Design review of the part built by this model. Coordinates are the model's own, in mm. A direction names the side the tool comes from. Coordinates: 2 decimals unless noted, no trailing zeros. Order: outer loops, then holes, each group sorted by start corner. A loop starts at its lowest first (then second) coordinate and runs counter-clockwise, first axis right, second up. Notation, with made-up numbers: M 48.25,20 L 57.25,20 A32 ccw 57.25,54 Z; hole C -36.5,-30.5 d9. An arc over 180 degrees is marked long. Answer in a Markdown table with one row per item.
from build123d import *

# Parameters (mm, degrees)
F_190_X_200_TRAY_FLOOR_SKETCH_W                       = 190
F_190_X_200_TRAY_FLOOR_SKETCH_H                       = 208
F_4_MM_TRAY_FLOOR_DEPTH                               = 4
ELECTRONICS_COMPARTMENT_WALL_SKETCH_W                 = 190
ELECTRONICS_COMPARTMENT_WALL_SKETCH_H                 = 175
ELECTRONICS_COMPARTMENT_WALL_SKETCH_W_2               = 176
ELECTRONICS_COMPARTMENT_WALL_SKETCH_H_2               = 161
F_22_MM_PERIMETER_WALLS_DEPTH                         = 22
F_3_2_START                                           = 17.2
EXTERNAL_WALL_CORD_GASKET_GROOVE_SKETCH_W             = 192
EXTERNAL_WALL_CORD_GASKET_GROOVE_SKETCH_H             = 177
EXTERNAL_WALL_CORD_GASKET_GROOVE_SKETCH_W_2           = 185.4
EXTERNAL_WALL_CORD_GASKET_GROOVE_SKETCH_H_2           = 170.4
F_3_2_HIGH_X_2_3_DEEP_EXTERNAL_PERIMETER_G_DEPTH      = 3.2
F_24_MM_GPS_ANTENNA_SHELF_SKETCH_W                    = 24
F_24_MM_GPS_ANTENNA_SHELF_SKETCH_H                    = 24
F_2_MM_GPS_ANTENNA_SHELF_DEPTH                        = 2
F_20_MM_GPS_ANTENNA_GUIDE_RING_SKETCH_W               = 24
F_20_MM_GPS_ANTENNA_GUIDE_RING_SKETCH_H               = 24
F_20_MM_GPS_ANTENNA_GUIDE_RING_SKETCH_W_2             = 20
F_20_MM_GPS_ANTENNA_GUIDE_RING_SKETCH_H_2             = 20
F_8_5_MM_GPS_ANTENNA_GUIDE_RING_DEPTH                 = 8.5
LEFT_GPS_ANTENNA_SNAP_LIP_SKETCH_W                    = 2.5
LEFT_GPS_ANTENNA_SNAP_LIP_SKETCH_H                    = 16
LEFT_GPS_ANTENNA_SNAP_LIP_DEPTH                       = 1.4
RIGHT_GPS_ANTENNA_SNAP_LIP_SKETCH_W                   = 2.5
RIGHT_GPS_ANTENNA_SNAP_LIP_SKETCH_H                   = 16
RIGHT_GPS_ANTENNA_SNAP_LIP_DEPTH                      = 1.4
F_190_MM_WIDE_ANGLED_DISPLAY_BULKHEAD_DEPTH           = 95
F_190_MM_WIDE_ANGLED_DISPLAY_BULKHEAD_DEPTH_BACK      = 95
F_92_X_58_MM_DISPLAY_OPENING_DEPTH                    = 46
F_92_X_58_MM_DISPLAY_OPENING_DEPTH_BACK               = 46
F_18_MM_FRONT_12_V_AND_SENSOR_HARNESS_PASS_DEPTH      = 40
F_18_MM_FRONT_12_V_AND_SENSOR_HARNESS_PASS_DEPTH_BACK = 40
F_18_MM_FRONT_HARNESS_GROMMET_SKETCH_R                = 9
LEFT_SCREEN_HOLDER_CORNER_CHAMFER_DEPTH               = 110
LEFT_SCREEN_HOLDER_CORNER_CHAMFER_DEPTH_BACK          = 110
RIGHT_SCREEN_HOLDER_CORNER_CHAMFER_DEPTH              = 110
RIGHT_SCREEN_HOLDER_CORNER_CHAMFER_DEPTH_BACK         = 110


with BuildPart() as part:
    # 190 x 200 Tray Floor Sketch → 4 mm Tray Floor (new body)
    with BuildSketch(Plane.XY):
        with Locations((0, 96)):
            Rectangle(F_190_X_200_TRAY_FLOOR_SKETCH_W, F_190_X_200_TRAY_FLOOR_SKETCH_H)
    extrude(amount=F_4_MM_TRAY_FLOOR_DEPTH)

    # Electronics Compartment Wall Sketch → 22 mm Perimeter Walls (add)
    with BuildSketch(Plane.XY):
        with Locations((0, 112.5)):
            Rectangle(ELECTRONICS_COMPARTMENT_WALL_SKETCH_W, ELECTRONICS_COMPARTMENT_WALL_SKETCH_H)
        with Locations((0, 112.5)):
            Rectangle(ELECTRONICS_COMPARTMENT_WALL_SKETCH_W_2, ELECTRONICS_COMPARTMENT_WALL_SKETCH_H_2, mode=Mode.SUBTRACT)
    extrude(amount=F_22_MM_PERIMETER_WALLS_DEPTH)

    # External Wall Cord Gasket Groove Sketch → 3.2 High x 2.3 Deep External Perimeter Gasket Groove (cut)
    with BuildSketch(Plane.XY.offset(F_3_2_START)):
        with Locations((0, 112.5)):
            Rectangle(EXTERNAL_WALL_CORD_GASKET_GROOVE_SKETCH_W, EXTERNAL_WALL_CORD_GASKET_GROOVE_SKETCH_H)
        with Locations((0, 112.5)):
            Rectangle(EXTERNAL_WALL_CORD_GASKET_GROOVE_SKETCH_W_2, EXTERNAL_WALL_CORD_GASKET_GROOVE_SKETCH_H_2, mode=Mode.SUBTRACT)
    extrude(amount=-F_3_2_HIGH_X_2_3_DEEP_EXTERNAL_PERIMETER_G_DEPTH, mode=Mode.SUBTRACT)

    # 24 mm GPS Antenna Shelf Sketch → 2 mm GPS Antenna Shelf (add)
    with BuildSketch(Plane.XY.offset(12)):
        with Locations((-76, 56)):
            Rectangle(F_24_MM_GPS_ANTENNA_SHELF_SKETCH_W, F_24_MM_GPS_ANTENNA_SHELF_SKETCH_H)
    extrude(amount=F_2_MM_GPS_ANTENNA_SHELF_DEPTH)

    # 20 mm GPS Antenna Guide Ring Sketch → 8.5 mm GPS Antenna Guide Ring (add)
    with BuildSketch(Plane.XY.offset(13.5)):
        with Locations((-76, 56)):
            Rectangle(F_20_MM_GPS_ANTENNA_GUIDE_RING_SKETCH_W, F_20_MM_GPS_ANTENNA_GUIDE_RING_SKETCH_H)
        with Locations((-76, 56)):
            Rectangle(F_20_MM_GPS_ANTENNA_GUIDE_RING_SKETCH_W_2, F_20_MM_GPS_ANTENNA_GUIDE_RING_SKETCH_H_2, mode=Mode.SUBTRACT)
    extrude(amount=F_8_5_MM_GPS_ANTENNA_GUIDE_RING_DEPTH)

    # Left GPS Antenna Snap Lip Sketch → Left GPS Antenna Snap Lip (add)
    with BuildSketch(Plane.XY.offset(20.4)):
        with Locations((-84.75, 56)):
            Rectangle(LEFT_GPS_ANTENNA_SNAP_LIP_SKETCH_W, LEFT_GPS_ANTENNA_SNAP_LIP_SKETCH_H)
    extrude(amount=LEFT_GPS_ANTENNA_SNAP_LIP_DEPTH)

    # Right GPS Antenna Snap Lip Sketch → Right GPS Antenna Snap Lip (add)
    with BuildSketch(Plane.XY.offset(20.4)):
        with Locations((-67.25, 56)):
            Rectangle(RIGHT_GPS_ANTENNA_SNAP_LIP_SKETCH_W, RIGHT_GPS_ANTENNA_SNAP_LIP_SKETCH_H)
    extrude(amount=RIGHT_GPS_ANTENNA_SNAP_LIP_DEPTH)

    # Angled Display Bulkhead Side Profile → 190 mm Wide Angled Display Bulkhead (add, two sides: drawn at the far end of the back side and taken through both)
    with BuildSketch(Plane(origin=(0, 0, 0), x_dir=(0, 0, -1), z_dir=(1, 0, 0)).offset(-F_190_MM_WIDE_ANGLED_DISPLAY_BULKHEAD_DEPTH_BACK)):
        Polygon((-2, 15), (-2, 21), (-100, 66), (-100, 60), align=None)
    extrude(amount=F_190_MM_WIDE_ANGLED_DISPLAY_BULKHEAD_DEPTH + F_190_MM_WIDE_ANGLED_DISPLAY_BULKHEAD_DEPTH_BACK)

    # 92 x 58 Display Opening Side Profile → 92 x 58 mm Display Opening (cut, two sides: drawn at the far end of the back side and taken through both)
    with BuildSketch(Plane(origin=(0, 0, 0), x_dir=(0, 0, -1), z_dir=(1, 0, 0)).offset(-F_92_X_58_MM_DISPLAY_OPENING_DEPTH_BACK)):
        Polygon((-28.2, 25), (-28.2, 35), (-80.8, 59.2), (-80.8, 49.2), align=None)
    extrude(amount=F_92_X_58_MM_DISPLAY_OPENING_DEPTH + F_92_X_58_MM_DISPLAY_OPENING_DEPTH_BACK, mode=Mode.SUBTRACT)

    # 18 mm Front Harness Grommet Sketch → 18 mm Front 12 V and Sensor Harness Passage (cut, two sides: drawn at the far end of the back side and taken through both)
    with BuildSketch(Plane(origin=(0, 0, 0), x_dir=(1, 0, 0), z_dir=(0, 1, 0)).offset(-F_18_MM_FRONT_12_V_AND_SENSOR_HARNESS_PASS_DEPTH_BACK)):
        with Locations(Location((0, -15, 0), (0, 0, 90))):
            Circle(F_18_MM_FRONT_HARNESS_GROMMET_SKETCH_R)
    extrude(amount=F_18_MM_FRONT_12_V_AND_SENSOR_HARNESS_PASS_DEPTH + F_18_MM_FRONT_12_V_AND_SENSOR_HARNESS_PASS_DEPTH_BACK, mode=Mode.SUBTRACT)

    # Left Screen Holder Corner Chamfer Sketch → Left Screen Holder Corner Chamfer (cut, two sides: drawn at the far end of the back side and taken through both)
    with BuildSketch(Plane(origin=(0, 0, 0), x_dir=(1, 0, 0), z_dir=(0, 1, 0)).offset(-LEFT_SCREEN_HOLDER_CORNER_CHAMFER_DEPTH_BACK)):
        Polygon((-95, -100), (-80, -100), (-95, -85), align=None)
    extrude(amount=LEFT_SCREEN_HOLDER_CORNER_CHAMFER_DEPTH + LEFT_SCREEN_HOLDER_CORNER_CHAMFER_DEPTH_BACK, mode=Mode.SUBTRACT)

    # Right Screen Holder Corner Chamfer Sketch → Right Screen Holder Corner Chamfer (cut, two sides: drawn at the far end of the back side and taken through both)
    with BuildSketch(Plane(origin=(0, 0, 0), x_dir=(1, 0, 0), z_dir=(0, 1, 0)).offset(-RIGHT_SCREEN_HOLDER_CORNER_CHAMFER_DEPTH_BACK)):
        Polygon((95, -100), (80, -100), (95, -85), align=None)
    extrude(amount=RIGHT_SCREEN_HOLDER_CORNER_CHAMFER_DEPTH + RIGHT_SCREEN_HOLDER_CORNER_CHAMFER_DEPTH_BACK, mode=Mode.SUBTRACT)


solid = part.part
(1) Add section D-D, the plane y = 84. Give the boundary of the cut face in (x, z).
Return value:
| item | result |
|---|---|
| outline | M -95,0 L 95,0 L 95,14 L 92.7,14 L 92.7,17.2 L 95,17.2 L 95,22 L 88,22 L 88,4 L -88,4 L -88,22 L -95,22 L -95,17.2 L -92.7,17.2 L -92.7,14 L -95,14 Z |
(2) Insertion check: pin 1 Ø1.4 at (x, z) = (-52, 15) entering from -Y; pin 2 Ø4 at (x, z) = (-45, 20) entering from -Y; pin 3 Ø9 at (x, z) = (-77.5, 17.5) entering from -Y; pin 4 Ø1.5 at (x, z) = (43.5, 43.5) entering from +Y. Each pin has a flat end and moves straight along its axis. Give the tip position at first contact, or say it passes through.
Return value:
| item | result |
|---|---|
| pin 1 | stops at y = 20.65 |
| pin 2 | stops at y = 22.35 |
| pin 3 | stops at y = 20.05 |
| pin 4 | passes through |
(3) Draft analysis for pull direction Y (two halves, no side actions). For faces 5 (the flat face through (-1, 54, 80.8)), 6 (the flat face through (-88, 111, 13)), 7 (the flat face through (-1.3, 25, 5.8)), 8 (the flat face through (-1.33, 52.96, 84.67)), state which applies: pulls with the +Y half, pulls with the -Y half, needs draft (parallel to the pull), parting line crosses it, or undercut.
Return value:
| item | result |
|---|---|
| face 5 | needs draft |
| face 6 | undercut |
| face 7 | undercut |
| face 8 | pulls with the -Y half |
(4) Add section C-C, the plane x = -58. Give the boundary of the cut face in (y, z), and give its area (3 significant figures).
Return value:
| item | result |
|---|---|
| outline | M -8,0 L 200,0 L 200,14 L 197.7,14 L 197.7,17.2 L 200,17.2 L 200,22 L 193,22 L 193,4 L 32,4 L 32,22 L 30.18,22 L 66,100 L 60,100 L 15.92,4 L -8,4 Z; hole M 21.92,4 L 25,4 L 25,10.71 Z; hole M 26.51,14 L 27.3,14 L 27.3,15.72 Z |
| area | 1,620 mm2 |
(5) For faces 1 (the flat face through (-1, 4, 4)), 2 (the flat face through (-46, 42, 55)), 3 (the flat face through (-76, 56, 12)), 4 (the flat face through (-1, 193, 13)), list the 3-axis set-ups (+Z, -Z, +X, -X, +Y, -Y) from which the entire face can be reached by the end or side of a thin tool; tool diameter is ignored.
Return value:
| item | result |
|---|---|
| face 1 | +Z, +X, -X, -Y |
| face 2 | +Y, -Y |
| face 3 | none |
| face 4 | +Z |
(6) For line 1 along X through (y, z) = (28.75, 15); line 2 along Y through (x, z) = (-77, 16); line 3 along Z through (x, y) = (0, 24), list the stretches that pass through material, from the lowest coordinate up. Write a range as from..to.
Return value:
| item | result |
|---|---|
| line 1 | x = -92.7..-9, 9..92.7 |
| line 2 | y = 21.43..32, 44..46, 66..68, 193..197.7 |
| line 3 | z = 0..4 |
(7) Add section A-A, the plane x = 27. Give the boundary of the cut face in (y, z).
Return value:
| item | result |
|---|---|
| outline | M -8,0 L 200,0 L 200,14 L 197.7,14 L 197.7,17.2 L 200,17.2 L 200,22 L 193,22 L 193,4 L 32,4 L 32,22 L 30.18,22 L 33.03,28.2 L 27.03,28.2 L 15.92,4 L -8,4 Z; M 51.18,80.8 L 57.18,80.8 L 66,100 L 60,100 Z; hole M 21.92,4 L 25,4 L 25,10.71 Z; hole M 26.51,14 L 27.3,14 L 27.3,15.72 Z |
(8) Add section B-B, the plane z = 55.5. Give the boundary of the cut face in (x, y).
Return value:
| item | result |
|---|---|
| outline | M -95,39.57 L -46,39.57 L -46,45.57 L -95,45.57 Z; M 46,39.57 L 95,39.57 L 95,45.57 L 46,45.57 Z |
